```python
from build123d import *

# Parameters (mm, degrees)
SKETCH_R      = 1.85
PAD_DEPTH     = 3
SKETCH812_R   = 2.85
PAD348_DEPTH  = 10
SKETCH813_R   = 3.513871
SKETCH813_R_2 = 3.587043
PAD349_DEPTH  = 4
SKETCH821_W   = 11.37968
SKETCH821_H   = 7.430097
PAD355_DEPTH  = 10
PAD363_DEPTH  = 6


with BuildPart() as part:
    # Sketch → Pad (new body)
    with BuildSketch(Plane.XZ):
        with BuildLine():
            Line((17.170527, 114.035013), (29.028223, 114.035013))
            ThreePointArc((34.420691, 109.455462), (32.565559, 112.735644), (29.028223, 114.035013))
            Line((34.420691, 109.455462), (41.249141, 67.851686))
            Line((41.249141, 67.851686), (44.41543, 58.566272))
            ThreePointArc((44.41543, 58.566272), (45.948377, 56.503803), (48.395228, 55.718549))
            Line((48.395228, 55.718549), (55.488024, 55.718549))
            ThreePointArc((59.596813, 51.60976), (58.393377, 54.515112), (55.488024, 55.718549))
            Line((59.596813, 51.60976), (59.596813, 41.694012))
            ThreePointArc((59.596813, 41.694012), (59.634099, 37.602359), (59.745945, 33.512064))
            Line((59.745945, 33.512064), (60.639802, 8.999999))
            Line((25, 8.999999), (60.639802, 8.999999))
            Line((28, 42), (25, 8.999999))
            Line((28, 42), (25.842674, 51.783651))
            ThreePointArc((24.578785, 63.385024), (24.89569, 57.550016), (25.842674, 51.783651))
            Line((24.578785, 63.385024), (24.578785, 74.280037))
            ThreePointArc((24.578785, 74.280037), (23.273536, 79.833608), (19.63109, 84.224328))
            Line((19.63109, 84.224328), (15.461415, 87.377315))
            ThreePointArc((12.16968, 94.057692), (13.023718, 90.327332), (15.461415, 87.377315))
            Line((12.16968, 94.057692), (12.286198, 109.188152))
            ThreePointArc((17.170527, 114.035013), (13.730006, 112.617656), (12.286198, 109.188152))
        make_face()
        with Locations((17.961559, 107.033859)):
            Circle(SKETCH_R, mode=Mode.SUBTRACT)
        with Locations((52.019562, 24.038517)):
            Circle(SKETCH_R, mode=Mode.SUBTRACT)
    extrude(amount=PAD_DEPTH)

    # Sketch812 → Pad348 (join)
    with BuildSketch(Plane.XY.offset(19)):
        with BuildLine():
            Line((35.385866, -0.616313), (31, -0.47951))
            Line((31, -0.47951), (24.245244, -0.47951))
            Line((24.245244, -0.47951), (17, -22))
            Line((17, -22), (18.714132, -22.779449))
            Line((18.714132, -22.779449), (20.699953, -23))
            Line((20.699953, -23), (26.461662, -26))
            Line((26.461662, -26), (28, -30.707495))
            Line((28, -30.707495), (27.531696, -36))
            Line((27.531696, -36), (25, -40.33778))
            Line((25, -40.33778), (20.617645, -43))
            Line((20.617645, -43), (16.419827, -43.712494))
            Line((16.419827, -43.712494), (12.22201, -41.737053))
            Line((12.22201, -41.737053), (10.684048, -40.962522))
            Line((10.684048, -40.962522), (8.352329, -49.76217))
            ThreePointArc((8.352329, -49.76217), (9.758834, -56.757072), (16.160124, -59.908323))
            Line((16.160124, -59.908323), (22.494802, -59.908323))
            ThreePointArc((22.494802, -59.908323), (23.211929, -59.71442), (23.733626, -59.185552))
            Line((23.733626, -59.185552), (33.781615, -41.410286))
            Line((42.205357, -35.669304), (33.781615, -41.410286))
            Line((42.271875, -26.390701), (42.205357, -35.669304))
            Line((42.271875, -26.390701), (56.841603, -0.616313))
            Line((56.841603, -0.616313), (35.385866, -0.616313))
        make_face()
        with Locations((17.460455, -55)):
            Circle(SKETCH812_R, mode=Mode.SUBTRACT)
    extrude(amount=-PAD348_DEPTH)

    # Sketch813 → Pad349 (join)
    with BuildSketch(Plane.XY.offset(90)):
        with BuildLine():
            Line((18.169887, -0.624235), (26.367772, -19.070229))
            ThreePointArc((27.333045, -21.643874), (26.888629, -20.342717), (26.367772, -19.070229))
            Line((27.333045, -21.643874), (28.631721, -25.850496))
            ThreePointArc((24.357214, -36.0031), (28.341536, -31.704461), (28.631721, -25.850496))
            Line((24.357214, -36.0031), (8.402813, -44.195061))
            ThreePointArc((8.402813, -44.195061), (4.422376, -47.325464), (1.905131, -51.719412))
            Line((1.905131, -51.719412), (1.74589, -52.187085))
            ThreePointArc((1.74589, -52.187085), (2.061173, -57.206378), (5.821391, -60.54606))
            Line((5.821391, -60.54606), (9.993196, -61.999858))
            ThreePointArc((9.993196, -61.999858), (12.851411, -61.847603), (14.782453, -59.734867))
            Line((14.782453, -59.734867), (16.394974, -55.344035))
            ThreePointArc((16.394974, -55.344035), (16.425444, -55.254007), (16.451264, -55.162537))
            Line((16.451264, -55.162537), (16.622268, -54.491485))
            ThreePointArc((26.49366, -49.560226), (20.430172, -49.768242), (16.622268, -54.491485))
            Line((26.49366, -49.560226), (28.791165, -50.517281))
            ThreePointArc((35.736479, -57.415769), (32.940269, -53.285486), (28.791165, -50.517281))
            Line((35.736479, -57.415769), (36.465842, -59.133842))
            ThreePointArc((36.465842, -59.133842), (40.075749, -62.413453), (44.914196, -61.799683))
            Line((44.914196, -61.799683), (46.318309, -60.923252))
            ThreePointArc((46.318309, -60.923252), (50.028994, -56.809581), (51.000403, -51.355423))
            Line((51.000403, -51.355423), (48.606712, -28.103775))
            ThreePointArc((48.606712, -28.103775), (47.070039, -20.895597), (44.031508, -14.180947))
            Line((44.031508, -14.180947), (36.044554, -0.624235))
            Line((36.044554, -0.624235), (18.169887, -0.624235))
        make_face()
        with Locations((8, -53.707806)):
            Circle(SKETCH813_R, mode=Mode.SUBTRACT)
        with Locations((41.795517, -53)):
            Circle(SKETCH813_R_2, mode=Mode.SUBTRACT)
    extrude(amount=PAD349_DEPTH)

    # Sketch821 → Pad355 (join)
    with BuildSketch(Plane.XZ):
        Polygon((22.156289, 112.186128), (27.568653, 112.186128), (27.568653, 94.657045), (30.525631, 85.906328), (35.012636, 65.899044), (42.218135, 54.723457), (56.839641, 54.774327), (59.23116, 41.91714), (58.653773, 37.89675), (44.278898, 37.89675), (41.369676, 26.918821), (52.806533, 14.952882), (49.043392, 10.924277), (37.294467, 24.947567), (40.651068, 40.30126), (36.476615, 54.317373), (28.98766, 65.755908), (22.156289, 91.93571), align=None)
        with Locations((49.397274, 46.051621)):
            Rectangle(SKETCH821_W, SKETCH821_H, mode=Mode.SUBTRACT)
    extrude(amount=PAD355_DEPTH)

    # Sketch840 → Pad363 (join)
    with BuildSketch(Plane.YZ.offset(35)):
        Polygon((-43.607986, 90.449928), (-38.696293, 90.449928), (-2.349776, 53.489452), (-2.104192, 47.349838), align=None)
        Polygon((-36.262971, 17.706057), (-30.339335, 17.706057), (-1.605939, 38.713028), (-2.09711, 43.133553), align=None)
    extrude(amount=PAD363_DEPTH)


solid = part.part
```
Could you check a few things on this model? Use its own coordinates, in mm. A direction names the side the tool comes from. Give positions to 0.01 mm unless a question says otherwise; leave off trailing zeros. Loops run counter-clockwise (first coordinate to the right, second up) from the corner with the lowest first, then second, coordinate; pieces in that order, holes last. Notation, with made-up numbers: (-21, 61) - (-2, 61) arc R10 ccw to (-2, 67) - close; hole circle Ø4 at (47, -11.75). An arc over 180 degrees is marked (long way). Answer in a Markdown table with one row per item. Add a question column.
Q1. We'd pull the mould along X, two halves only. Please class faces 4 (the face through (19, -59.908, 14)), 5 (the face through (35, -22, 71)), 6 (the face through (20.51, -49.73, 91.97)): +X half, -X half, draft (parallel to the pull), parting line (faces both ways), or undercut.
Q2. If we section it at B-B (z = 96): List the corners of the cut face in (x, y) for me.
Q3. For pin 1 (10 mm diameter, centred on x = 20.5, z = 100.5, fed in from -Y); pin 2 (2 mm diameter, centred on x = 37.5, z = 42.5, fed in from -Y); pin 3 (3.5 mm diameter, centred on x = 52.02, z = 24.04, fed in from -Y); pin 4 (2.5 mm diameter, centred on x = 51, y = -1, fed in from +Z), each with a flat end and sliding along its axis, tell me the tip position at first contact or that it passes through.
Q4. Which directions (+Z, -Z, +X, -X, +Y, -Y) give clear straight access to the entire face, cutting with the end or side of a thin tool? Please do faces 1 (the face through (38.565, -6.451, 60.389)), 2 (the face through (9.535, -45.301, 14.07)), 3 (the face through (49, -6, 49.767)).
Q5. Please list where these lines run through material, in increasing order: L1, parallel to Z at x = 40.5, y = -12; L2, parallel to Z at x = 22.5, y = -56.5; L3, parallel to Y at x = 14.5, z = 89. Write a range as from..to.
Q6. If we section it at A-A (y = -17): List the corners of the cut face in (x, z) for me, plus the area to 3 significant figures.
The answers:
| question | item | result |
|---|---|---|
| 1 | face 4 | draft |
| 1 | face 5 | -X half |
| 1 | face 6 | undercut |
| 2 | outline | (12.18, -3) - (22.16, -3) - (22.16, -10) - (27.57, -10) - (27.57, -3) - (36.63, -3) - (36.63, 0) - (12.18, 0) - close |
| 3 | pin 1 | stops at y = -10 |
| 3 | pin 2 | stops at y = -4.29 |
| 3 | pin 3 | passes through |
| 3 | pin 4 | stops at z = 55.72 |
| 4 | face 1 | +X |
| 4 | face 2 | -Z, -X, +Y |
| 4 | face 3 | -Y |
| 5 | L1 | z = 9..19, 31.11..35.76, 57.63..63.3, 90..94 |
| 5 | L2 | z = 9..19 |
| 5 | L3 | y = -3..0 |
| 6 | outline | (18.68, 9) - (47.58, 9) - (47.58, 19) - (18.68, 19) - close; (25.45, 90) - (45.52, 90) - (45.52, 94) - (25.45, 94) - close; (35, 27.46) - (41, 27.46) - (41, 32.04) - (35, 32.04) - close; (35, 62.82) - (41, 62.82) - (41, 68.39) - (35, 68.39) - close |
| 6 | area | 430 mm^2 |
